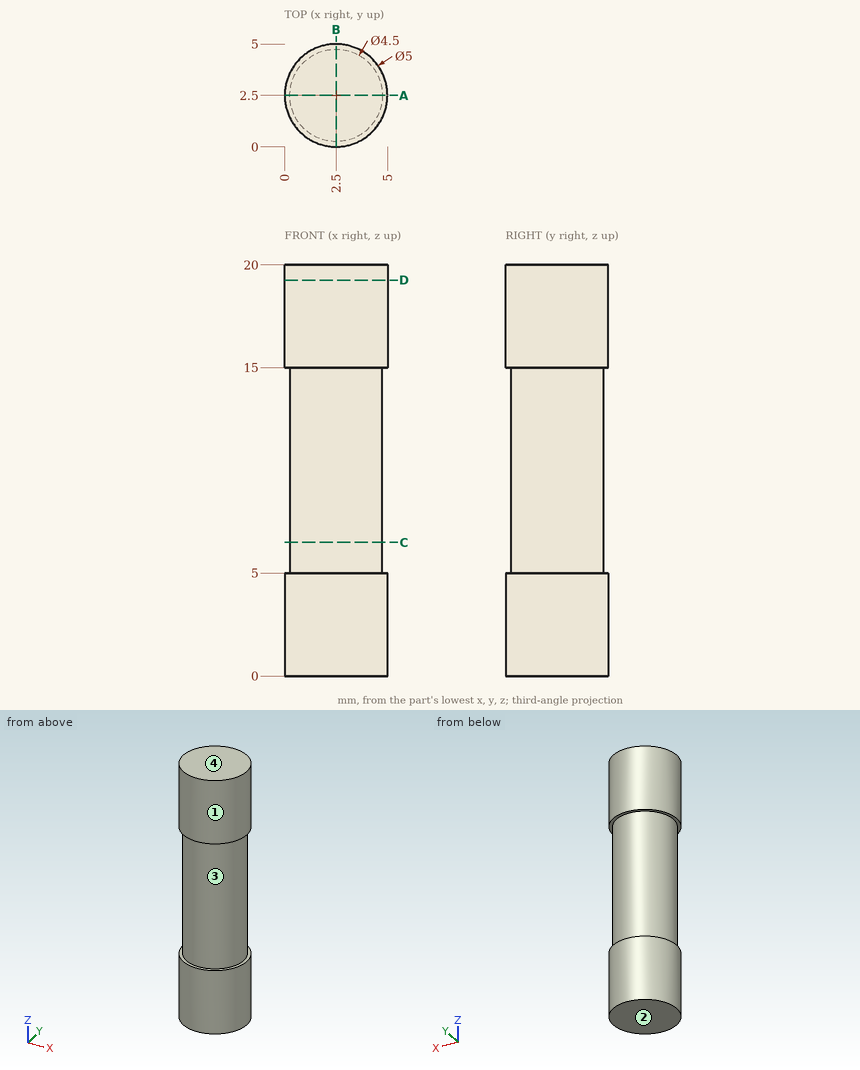
Answer from the drawing. Dimensions are ordinates in mm from the lowest x, y and z of the part. Coordinates: 2 decimals unless noted, no trailing zeros. Write each loop counter-clockwise with the first axis right and the second up, starting at its lowest first coordinate (ties: lowest second). Pieces come first, ordered by that corner, then holes. Notation, with made-up numbers: M 71.25,-6.75 L 77.25,-6.75 A23 ccw 77.25,18.25 Z; hole C 61,45 d2. An arc over 180 degrees is marked long. Write item = value, one per line.
1. The part is cut by section C-C (z = 6.5). Determine the outline of the cut face in (x, y), then the cut area to 3 significant figures.
Solution:
outline = C 2.5,2.5 d4.5
area = 15.9 mm2
2. Flat-ended cylindrical pins translate along their axes: pin 1 (3 mm diameter, centred on x = 1, z = 17, fed in from -Y); pin 2 (2 mm diameter, centred on y = 1, z = 9.5, fed in from -X). Find the tip coordinate at first contact, or state that the pin passes through.
Solution:
pin_1 = 0
pin_2 = 0.31
3. The part is cut by section D-D (z = 19.25). Determine the outline of the cut face in (x, y), then the cut area to 3 significant figures.
Solution:
outline = C 2.5,2.5 d5
area = 19.6 mm2
4. Straight lines are drawn through the part: line 1 (Z direction, x = 4.1, y = 4.3); line 2 (X direction, y = 2.6, z = 11.75); line 3 (Y direction, x = 2.65, z = 10.75) (3 decimals). For each, find the intervals that lie inside material, in ascending order. Write a range as from..to.
Solution:
line_1 = 0..5, 15..20
line_2 = 0.25..4.75
line_3 = 0.255..4.745
5. Determine the mould class of the marked faces 1, 2, 3 and 4 for opening direction Z: released by +Z, released by -Z, zero draft, split by the parting line, or undercut.
Solution:
face_1 = zero draft
face_2 = released by -Z
face_3 = undercut
face_4 = released by +Z
6. The part is cut by section A-A (y = 2.5). Determine the outline of the cut face in (x, z).
Solution:
outline = M 0,0 L 5,0 L 5,5 L 4.75,5 L 4.75,15 L 5,15 L 5,20 L 0,20 L 0,15 L 0.25,15 L 0.25,5 L 0,5 Z
